```python
from build123d import *

# Parameters (mm, degrees)
PAD_DEPTH    = 7
SKETCH001_R  = 1.5
POCKET_DEPTH = 13.501


with BuildPart() as part:
    # Sketch → Pad (new body)
    with BuildSketch(Plane.XY):
        with BuildLine():
            ThreePointArc((-1.5, 4.242641), (0, -4.5), (1.5, 4.242641))
            Line((1.5, 4.242641), (1.5, 12.809475))
            Line((1.5, 12.809475), (5.5, 12.809475))
            Line((5.5, 12.809475), (5.5, 5.809475))
            ThreePointArc((-5.5, 5.809475), (0, -8), (5.5, 5.809475))
            Line((-5.5, 5.809475), (-5.5, 12.809475))
            Line((-5.5, 12.809475), (-1.5, 12.809475))
            Line((-1.5, 12.809475), (-1.5, 4.242641))
        make_face()
    extrude(amount=PAD_DEPTH)

    # Sketch001 (on Face7 of Pad) → Pocket (cut, through all)
    with BuildSketch(Plane.YZ.offset(5.5)):
        with Locations((9.25, 3.5)):
            Circle(SKETCH001_R)
    extrude(amount=-POCKET_DEPTH, mode=Mode.SUBTRACT)


solid = part.part
```
Can you work these out from the model? Positions are in its coordinate system, mm. A direction names the side the tool comes from. Coordinates: 2 decimals unless noted, no trailing zeros. Loops run counter-clockwise (first coordinate to the right, second up) from the corner with the lowest first, then second, coordinate; pieces in that order, holes last. Notation, with made-up numbers: (19.5, 58.25) - (55.5, 58.25) arc R32 cw to (55.5, 91.25) - close; hole circle Ø1 at (23, 62.25). An arc over 180 degrees is marked (long way). Use a Markdown table: item, result.
Item 1: I want a section at A-A on z = 3.5. Please give me the cut outline in (x, y).
Numbers:
| item | result |
|---|---|
| outline | (-5.5, 5.81) arc R8 ccw (long way) to (5.5, 5.81) - (5.5, 7.75) - (1.5, 7.75) - (1.5, 4.24) arc R4.5 cw (long way) to (-1.5, 4.24) - (-1.5, 7.75) - (-5.5, 7.75) - close; (-5.5, 10.75) - (-1.5, 10.75) - (-1.5, 12.81) - (-5.5, 12.81) - close; (1.5, 10.75) - (5.5, 10.75) - (5.5, 12.81) - (1.5, 12.81) - close |
Item 2: Will these pins go through, and if not, where does the flat tip stop? pin 1 (3.5 mm diameter, centred on y = 8.5, z = 4, fed in from +X); pin 2 (4 mm diameter, centred on x = -4, z = 5.5, fed in from -Y).
Numbers:
| item | result |
|---|---|
| pin 1 | stops at x = 5.5 |
| pin 2 | stops at y = -7.75 |
Item 3: We'd pull the mould along Y, two halves only. Please class faces 6 (the face through (3, 12.809, 3)), 7 (the face through (1.5, 7.5, 3.5)), 8 (the face through (-3.47, 7.75, 3.57)), 9 (the face through (-0.176, -4.497, 3.451)): released by +Y, released by -Y, zero draft, split by the parting line, or undercut.
Numbers:
| item | result |
|---|---|
| face 6 | released by +Y |
| face 7 | zero draft |
| face 8 | undercut |
| face 9 | undercut |
Item 4: I want a section at C-C on x = 2.75. Please give me the cut outline in (y, z), and give its area (3 significant figures).
Numbers:
| item | result |
|---|---|
| outline | (-7.51, 0) - (-3.56, 0) - (-3.56, 7) - (-7.51, 7) - close; (3.56, 0) - (12.81, 0) - (12.81, 7) - (3.56, 7) - close; hole circle Ø3 at (9.25, 3.5) |
| area | 85.3 mm2 |
Item 5: I want a section at B-B on y = 6.25. Please give me the cut outline in (x, z), and give its area (3 significant figures).
Numbers:
| item | result |
|---|---|
| outline | (-5.5, 0) - (-1.5, 0) - (-1.5, 7) - (-5.5, 7) - close; (1.5, 0) - (5.5, 0) - (5.5, 7) - (1.5, 7) - close |
| area | 56.0 mm2 |
Item 6: If I drill on probe 1 along Z at (x, y) = (-2.5, 9.25); probe 2 along X at (y, z) = (8.75, 6); probe 3 along Y at (x, z) = (-3.5, 4.25), over which ranges is the centre line in solid material (lowest first)? Write a range as from..to.
Numbers:
| item | result |
|---|---|
| probe 1 | z = 0..2, 5..7 |
| probe 2 | x = -5.5..-1.5, 1.5..5.5 |
| probe 3 | y = -7.19..-2.83, 2.83..7.95, 10.55..12.81 |
Item 7: For faces 1 (the face through (-1.5, 7.6, 3.5)), 2 (the face through (5.5, 11, 3)), 3 (the face through (3.53, 7.75, 3.57)), 4 (the face through (2, 5, 0)), 5 (the face through (-5.5, 11, 3)), which set-ups out of +Z, -Z, +X, -X, +Y, -Y let a thin tool reach every point of the face, with its end or its side?
Numbers:
| item | result |
|---|---|
| face 1 | +Z, -Z, +Y |
| face 2 | +Z, -Z, +X, +Y |
| face 3 | +X, -X |
| face 4 | -Z, +X, -X, +Y, -Y |
| face 5 | +Z, -Z, -X, +Y |
Item 8: I want a section at D-D on y = 9.25. Please give me the cut outline in (x, z).
Numbers:
| item | result |
|---|---|
| outline | (-5.5, 0) - (-1.5, 0) - (-1.5, 2) - (-5.5, 2) - close; (-5.5, 5) - (-1.5, 5) - (-1.5, 7) - (-5.5, 7) - close; (1.5, 0) - (5.5, 0) - (5.5, 2) - (1.5, 2) - close; (1.5, 5) - (5.5, 5) - (5.5, 7) - (1.5, 7) - close |
